```python
from build123d import *

# Parameters (mm, degrees)
SKETCH1_W            = 48
SKETCH1_H            = 53
BOSS_EXTRUDE1_DEPTH  = 10
SKETCH2_W            = 48
SKETCH2_H            = 5.616325
BOSS_EXTRUDE2_DEPTH  = 33.1917878
SKETCH4_W            = 4
SKETCH4_H            = 10
BOSS_EXTRUDE4_DEPTH  = 40
SKETCH5_W            = 48
SKETCH5_H            = 10.8609375
BOSS_EXTRUDE5_DEPTH  = 23.1917878
SKETCH6_W            = 48
SKETCH6_H            = 5
BOSS_EXTRUDE6_DEPTH  = 42.3
SKETCH7_W            = 12.8082122
SKETCH7_H            = 16.4772625
BOSS_EXTRUDE7_DEPTH  = 48
CUT_EXTRUDE1_REACH   = 84.426
SKETCH8_R            = 11.5
SKETCH8_R_2          = 1.5
FILLET1_R            = 10
FILLET2_R            = 4
SKETCH9_W            = 5
SKETCH9_H            = 16.4772625
BOSS_EXTRUDE9_DEPTH  = 48
CUT_EXTRUDE2_DEPTH   = 88.252507127
SKETCH11_W           = 51
SKETCH11_H           = 16.4772625
BOSS_EXTRUDE10_DEPTH = 49.45
BOSS_EXTRUDE11_DEPTH = 46
SKETCH16_W           = 47.95
SKETCH16_H           = 51
BOSS_EXTRUDE14_DEPTH = 2.55
SKETCH14_W           = 5
SKETCH14_H           = 42.3
BOSS_EXTRUDE13_DEPTH = 1.5
SKETCH17_W           = 51
SKETCH17_H           = 19.0272625
BOSS_EXTRUDE15_DEPTH = 9
BOSS_EXTRUDE16_DEPTH = 25
SKETCH19_R           = 1.9304
CUT_EXTRUDE3_DEPTH   = 125.404890183
CUT_EXTRUDE4_REACH   = 129.391


with BuildPart() as part:
    # Sketch1 → Boss-Extrude1 (new body)
    with BuildSketch(Plane.XY):
        with Locations((24, 26.5)):
            Rectangle(SKETCH1_W, SKETCH1_H)
    extrude(amount=BOSS_EXTRUDE1_DEPTH)

    # Sketch2 → Boss-Extrude2 (add)
    with BuildSketch(Plane(origin=(0, 0, 0), x_dir=(-1, 0, 0), z_dir=(0, 0, -1))):
        with Locations((-24, -2.8081625)):
            Rectangle(SKETCH2_W, SKETCH2_H)
    extrude(amount=-BOSS_EXTRUDE2_DEPTH)

    # Sketch4 → Boss-Extrude4 (add)
    with BuildSketch(Plane.XY.offset(10)):
        with Locations((2, 48)):
            Rectangle(SKETCH4_W, SKETCH4_H)
        with Locations((46, 48)):
            Rectangle(SKETCH4_W, SKETCH4_H)
    extrude(amount=BOSS_EXTRUDE4_DEPTH)

    # Sketch5 → Boss-Extrude5 (add)
    with BuildSketch(Plane.XY.offset(10)):
        with Locations((24, 5.43046875)):
            Rectangle(SKETCH5_W, SKETCH5_H)
    extrude(amount=BOSS_EXTRUDE5_DEPTH)

    # Sketch6 → Boss-Extrude6 (add)
    with BuildSketch(Plane.XZ.offset(5.616325)):
        with Locations((24, 30.6917878)):
            Rectangle(SKETCH6_W, SKETCH6_H)
    extrude(amount=BOSS_EXTRUDE6_DEPTH)

    # Sketch7 → Boss-Extrude7 (add)
    with BuildSketch(Plane.ZY):
        with Locations((-6.4041061, 2.62230625)):
            Rectangle(SKETCH7_W, SKETCH7_H)
    extrude(amount=-BOSS_EXTRUDE7_DEPTH)

    # Sketch8 → Cut-Extrude1 (cut, up to next)
    with BuildSketch(Plane(origin=(0, 0, 28.1917878), x_dir=(-1, 0, 0), z_dir=(0, 0, -1)), mode=Mode.PRIVATE) as cut_extrude1_sk1:
        with Locations((-24, -26.616325)):
            Circle(SKETCH8_R)
    cut_extrude1_tool1 = extrude(cut_extrude1_sk1.sketch, amount=-CUT_EXTRUDE1_REACH, mode=Mode.PRIVATE) & part.part
    # Sketch8 → Cut-Extrude1 (cut, up to next)
    with BuildSketch(Plane(origin=(0, 0, 28.1917878), x_dir=(-1, 0, 0), z_dir=(0, 0, -1)), mode=Mode.PRIVATE) as cut_extrude1_sk2:
        with Locations((-39.5, -11.116325)):
            Circle(SKETCH8_R_2)
    cut_extrude1_tool2 = extrude(cut_extrude1_sk2.sketch, amount=-CUT_EXTRUDE1_REACH, mode=Mode.PRIVATE) & part.part
    # Sketch8 → Cut-Extrude1 (cut, up to next)
    with BuildSketch(Plane(origin=(0, 0, 28.1917878), x_dir=(-1, 0, 0), z_dir=(0, 0, -1)), mode=Mode.PRIVATE) as cut_extrude1_sk3:
        with Locations((-39.5, -42.116325)):
            Circle(SKETCH8_R_2)
    cut_extrude1_tool3 = extrude(cut_extrude1_sk3.sketch, amount=-CUT_EXTRUDE1_REACH, mode=Mode.PRIVATE) & part.part
    # Sketch8 → Cut-Extrude1 (cut, up to next)
    with BuildSketch(Plane(origin=(0, 0, 28.1917878), x_dir=(-1, 0, 0), z_dir=(0, 0, -1)), mode=Mode.PRIVATE) as cut_extrude1_sk4:
        with Locations((-8.5, -11.116325)):
            Circle(SKETCH8_R_2)
    cut_extrude1_tool4 = extrude(cut_extrude1_sk4.sketch, amount=-CUT_EXTRUDE1_REACH, mode=Mode.PRIVATE) & part.part
    # Sketch8 → Cut-Extrude1 (cut, up to next)
    with BuildSketch(Plane(origin=(0, 0, 28.1917878), x_dir=(-1, 0, 0), z_dir=(0, 0, -1)), mode=Mode.PRIVATE) as cut_extrude1_sk5:
        with Locations((-8.5, -42.116325)):
            Circle(SKETCH8_R_2)
    cut_extrude1_tool5 = extrude(cut_extrude1_sk5.sketch, amount=-CUT_EXTRUDE1_REACH, mode=Mode.PRIVATE) & part.part
    add(cut_extrude1_tool1.solids().sort_by_distance((24, -26.616325, 28.191788))[0], mode=Mode.SUBTRACT)
    add(cut_extrude1_tool2.solids().sort_by_distance((39.5, -11.116325, 28.191788))[0], mode=Mode.SUBTRACT)
    add(cut_extrude1_tool3.solids().sort_by_distance((39.5, -42.116325, 28.191788))[0], mode=Mode.SUBTRACT)
    add(cut_extrude1_tool4.solids().sort_by_distance((8.5, -11.116325, 28.191788))[0], mode=Mode.SUBTRACT)
    add(cut_extrude1_tool5.solids().sort_by_distance((8.5, -42.116325, 28.191788))[0], mode=Mode.SUBTRACT)

    # Fillet1
    fillet1_edges = [part.edges().sort_by_distance(p)[0] for p in [
        (24, 10.8609375, 0),
    ]]
    fillet(fillet1_edges, radius=FILLET1_R)

    # Fillet2
    fillet2_edges = [part.edges().sort_by_distance(p)[0] for p in [
        (2, 43, 10),
        (46, 43, 10),
    ]]
    fillet(fillet2_edges, radius=FILLET2_R)

    # Sketch9 → Boss-Extrude9 (add)
    with BuildSketch(Plane(origin=(48, 0, 0), x_dir=(0, 0, -1), z_dir=(1, 0, 0))):
        with Locations((15.3082122, 2.62230625)):
            Rectangle(SKETCH9_W, SKETCH9_H)
    extrude(amount=-BOSS_EXTRUDE9_DEPTH)

    # Sketch10 → Cut-Extrude2 (cut, through all)
    with BuildSketch(Plane(origin=(48, 0, 0), x_dir=(0, 0, -1), z_dir=(1, 0, 0))):
        Polygon((17.8082122, 10.8609375), (-33.1917878, 10.8609375), (-76.887145623, 43.902095521), (-50.794096938, 74.436514195), (27.207463492, 71.105486703), align=None)
    extrude(amount=-CUT_EXTRUDE2_DEPTH, mode=Mode.SUBTRACT)

    # Sketch11 → Boss-Extrude10 (add)
    with BuildSketch(Plane(origin=(48, 0, 0), x_dir=(0, 0, -1), z_dir=(1, 0, 0))):
        with Locations((-7.6917878, 2.62230625)):
            Rectangle(SKETCH11_W, SKETCH11_H)
    extrude(amount=BOSS_EXTRUDE10_DEPTH)

    # Sketch12 → Boss-Extrude11 (add)
    with BuildSketch(Plane(origin=(0, 0, 28.1917878), x_dir=(-1, 0, 0), z_dir=(0, 0, -1))):
        Polygon((-48, -47.916325), (-45, -47.916325), (-45, -5.616325), (-49.5, -5.616325), (-49.5, -47.916325), align=None)
    extrude(amount=BOSS_EXTRUDE11_DEPTH)

    # Sketch16 → Boss-Extrude14 (add)
    with BuildSketch(Plane.XZ.offset(5.616325)):
        with Locations((73.475, 7.6917878)):
            Rectangle(SKETCH16_W, SKETCH16_H)
    extrude(amount=BOSS_EXTRUDE14_DEPTH)

    # Sketch14 → Boss-Extrude13 (add)
    with BuildSketch(Plane(origin=(49.5, 0, 0), x_dir=(0, 0, -1), z_dir=(1, 0, 0))):
        with Locations((-30.6917878, -26.766325)):
            Rectangle(SKETCH14_W, SKETCH14_H)
    extrude(amount=-BOSS_EXTRUDE13_DEPTH)

    # Sketch17 → Boss-Extrude15 (add)
    with BuildSketch(Plane(origin=(97.45, 0, 0), x_dir=(0, 0, -1), z_dir=(1, 0, 0))):
        with Locations((-7.6917878, 1.34730625)):
            Rectangle(SKETCH17_W, SKETCH17_H)
    extrude(amount=BOSS_EXTRUDE15_DEPTH)

    # Sketch18 → Boss-Extrude16 (add)
    with BuildSketch(Plane.XZ.offset(8.166325)):
        Polygon((49.5, -17.8082122), (106.45, -17.8082122), (106.45, -9.8082122), (106.45, 33.1917878), (97.45, 33.1917878), (97.45, -9.8082122), (49.5, -9.8082122), align=None)
    extrude(amount=BOSS_EXTRUDE16_DEPTH)

    # Sketch19 → Cut-Extrude3 (cut, through all)
    with BuildSketch(Plane.XY.offset(-9.8082122)):
        with Locations((58.475, -26.166325)):
            Circle(SKETCH19_R)
        with Locations((88.475, -26.166325)):
            Circle(SKETCH19_R)
    extrude(amount=-CUT_EXTRUDE3_DEPTH, mode=Mode.SUBTRACT)

    # Sketch20 → Cut-Extrude4 (cut, up to next)
    with BuildSketch(Plane.XY.offset(33.1917878), mode=Mode.PRIVATE) as cut_extrude4_sk1:
        with BuildLine():
            Line((7.184805756, -11.837618352), (7.433777419, -12.319738309))
            ThreePointArc((7.433777419, -12.319738309), (8.5, -12.969130092), (9.566222581, -12.319738309))
            Line((9.566222581, -12.319738309), (9.815194244, -11.837618352))
            ThreePointArc((9.815194244, -11.837618352), (8.5, -12.616325), (7.184805756, -11.837618352))
        make_face()
    cut_extrude4_tool1 = extrude(cut_extrude4_sk1.sketch, amount=-CUT_EXTRUDE4_REACH, mode=Mode.PRIVATE) & part.part
    # Sketch20 → Cut-Extrude4 (cut, up to next)
    with BuildSketch(Plane.XY.offset(33.1917878), mode=Mode.PRIVATE) as cut_extrude4_sk2:
        with BuildLine():
            Line((7.184805756, -42.837618352), (7.433777419, -43.319738309))
            ThreePointArc((7.433777419, -43.319738309), (8.5, -43.969130092), (9.566222581, -43.319738309))
            Line((9.566222581, -43.319738309), (9.815194244, -42.837618352))
            ThreePointArc((9.815194244, -42.837618352), (8.5, -43.616325), (7.184805756, -42.837618352))
        make_face()
    cut_extrude4_tool2 = extrude(cut_extrude4_sk2.sketch, amount=-CUT_EXTRUDE4_REACH, mode=Mode.PRIVATE) & part.part
    # Sketch20 → Cut-Extrude4 (cut, up to next)
    with BuildSketch(Plane.XY.offset(33.1917878), mode=Mode.PRIVATE) as cut_extrude4_sk3:
        with BuildLine():
            Line((38.184805756, -42.837618352), (38.433777419, -43.319738309))
            ThreePointArc((38.433777419, -43.319738309), (39.5, -43.969130092), (40.566222581, -43.319738309))
            Line((40.566222581, -43.319738309), (40.815194244, -42.837618352))
            ThreePointArc((40.815194244, -42.837618352), (39.5, -43.616325), (38.184805756, -42.837618352))
        make_face()
    cut_extrude4_tool3 = extrude(cut_extrude4_sk3.sketch, amount=-CUT_EXTRUDE4_REACH, mode=Mode.PRIVATE) & part.part
    # Sketch20 → Cut-Extrude4 (cut, up to next)
    with BuildSketch(Plane.XY.offset(33.1917878), mode=Mode.PRIVATE) as cut_extrude4_sk4:
        with BuildLine():
            Line((38.184805756, -11.837618352), (38.433777419, -12.319738309))
            ThreePointArc((38.433777419, -12.319738309), (39.5, -12.969130092), (40.566222581, -12.319738309))
            Line((40.566222581, -12.319738309), (40.815194244, -11.837618352))
            ThreePointArc((40.815194244, -11.837618352), (39.5, -12.616325), (38.184805756, -11.837618352))
        make_face()
    cut_extrude4_tool4 = extrude(cut_extrude4_sk4.sketch, amount=-CUT_EXTRUDE4_REACH, mode=Mode.PRIVATE) & part.part
    # Sketch20 → Cut-Extrude4 (cut, up to next)
    with BuildSketch(Plane.XY.offset(33.1917878), mode=Mode.PRIVATE) as cut_extrude4_sk5:
        with BuildLine():
            Line((19.405287598, -37.158555217), (24, -39.787183437))
            Line((24, -39.787183437), (28.594712402, -37.158555217))
            ThreePointArc((28.594712402, -37.158555217), (24, -38.116325), (19.405287598, -37.158555217))
        make_face()
    cut_extrude4_tool5 = extrude(cut_extrude4_sk5.sketch, amount=-CUT_EXTRUDE4_REACH, mode=Mode.PRIVATE) & part.part
    add(cut_extrude4_tool1.solids().sort_by_distance((8.5, -12.63481, 33.191788))[0], mode=Mode.SUBTRACT)
    add(cut_extrude4_tool2.solids().sort_by_distance((8.5, -43.63481, 33.191788))[0], mode=Mode.SUBTRACT)
    add(cut_extrude4_tool3.solids().sort_by_distance((39.5, -43.63481, 33.191788))[0], mode=Mode.SUBTRACT)
    add(cut_extrude4_tool4.solids().sort_by_distance((39.5, -12.63481, 33.191788))[0], mode=Mode.SUBTRACT)
    add(cut_extrude4_tool5.solids().sort_by_distance((24, -38.507203, 33.191788))[0], mode=Mode.SUBTRACT)


solid = part.part
```
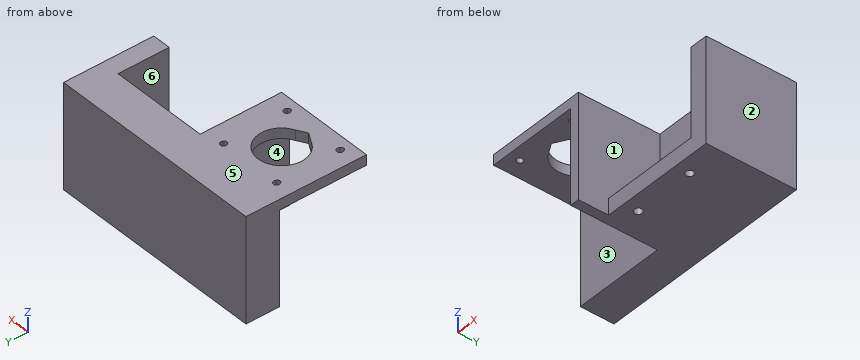
Verification items for the finished model (mm, model axes). Face numbers are marked on the shaded views. A direction names the side the tool comes from. Give positions to 0.01 mm unless a question says otherwise; leave off trailing zeros. Write each loop counter-clockwise with the first axis right and the second up, starting at its lowest first coordinate (ties: lowest second). Pieces come first, ordered by that corner, then holes. Notation, with made-up numbers: M 50.5,-8.75 L 76.5,-8.75 A29 ccw 76.5,13.25 Z; hole C 15,63.25 d2. An arc over 180 degrees is marked long. One line per question, with ' | ' between items.
1) Gauge pin test, flat ends, axial feed: pin 1 Ø3.5 at (x, y) = (39.5, -11.12) entering from +Z; pin 2 Ø12.5 at (y, z) = (-20.5, -5.5) entering from -X; pin 3 Ø15.5 at (x, z) = (87, 4.5) entering from -Y; pin 4 Ø3.5 at (x, y) = (88.48, -26.17) entering from +Z. Record the tip position at first contact, or that the pin passes through.
Result:
pin 1: stops at z = 33.19 | pin 2: stops at x = 45 | pin 3: stops at y = -8.17 | pin 4: passes through
2) Set-up check for the marked faces 1, 2 and 3: record each of +Z, -Z, +X, -X, +Y, -Y from which the full face is reachable in a straight line by a thin tool's end or side.
Result:
face 1: +Z, -Y | face 2: +Z, -Z, +X, +Y, -Y | face 3: -Z, -X, -Y
3) Section check C-C on z = 14.5. Enter the section's corners in (x, y), plus the area to 3 significant figures.
Result:
outline: M 0,-5.62 L 45,-5.62 L 45,-47.92 L 49.5,-47.92 L 49.5,-8.17 L 97.45,-8.17 L 97.45,-33.17 L 106.45,-33.17 L 106.45,10.86 L 0,10.86 Z | area: 2,310 mm2
4) Thickness scan on line 1 along Y through (x, z) = (39.5, 31.7); line 2 along X through (y, z) = (-26, 5); line 3 along X through (y, z) = (-32.5, 31). Record the ranges inside material, lowest first. Write a range as [from, to].
Result:
line 1: y = [-47.92, -43.97], [-40.62, -12.97], [-9.62, 10.86] | line 2: x = [45, 49.5], [97.45, 106.45] | line 3: x = [0, 14.12], [33.88, 49.5], [97.45, 106.45]
5) Section check B-B on x = 88. Enter the section's corners in (y, z).
Result:
outline: M -33.17,-17.81 L -28.04,-17.81 L -28.04,-9.81 L -33.17,-9.81 Z; M -24.3,-17.81 L 10.86,-17.81 L 10.86,33.19 L -8.17,33.19 L -8.17,-9.81 L -24.3,-9.81 Z
6) Mould release check, pull along X, two halves, no side actions. Record for the marked faces 4, 5 and 6: released by +X, released by -X, zero draft, split by the parting line, or undercut.
Result:
face 4: released by -X | face 5: zero draft | face 6: undercut
7) Section check D-D on x = 14. Enter the section's corners in (y, z), plus the area to 3 significant figures.
Result:
outline: M -47.92,28.19 L -32.3,28.19 L -32.3,33.19 L -47.92,33.19 Z; M -20.94,28.19 L -5.62,28.19 L -5.62,-17.81 L 10.86,-17.81 L 10.86,33.19 L -20.94,33.19 Z | area: 995 mm2
8) Section check A-A on x = 39.5. Enter the section's corners in (y, z), plus the area to 3 significant figures.
Result:
outline: M -47.92,28.19 L -43.97,28.19 L -43.97,33.19 L -47.92,33.19 Z; M -40.62,28.19 L -12.97,28.19 L -12.97,33.19 L -40.62,33.19 Z; M -9.62,28.19 L -5.62,28.19 L -5.62,-17.81 L 10.86,-17.81 L 10.86,33.19 L -9.62,33.19 Z | area: 1,020 mm2
